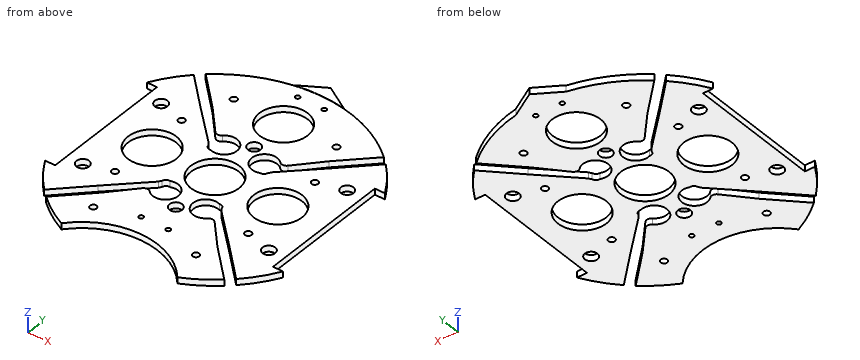
```python
from build123d import *

# Parameters (mm, degrees)
BOSS_EXTRUDE2_DEPTH      = 3.048
SKETCH4_R                = 38.1
CUT_EXTRUDE3_DEPTH       = 4.048
BOSS_EXTRUDE3_DEPTH      = 3.175
SKETCH12_R               = 1.143
CUT_EXTRUDE9_DEPTH       = 4.175
SKETCH15_R               = 1.651
CUT_EXTRUDE12_DEPTH      = 75.692
SKETCH17_R               = 1.651
CUT_EXTRUDE14_DEPTH      = 97.79
SKETCH18_R               = 12.192
CUT_EXTRUDE15_DEPTH      = 35.56
SKETCH19_R               = 3.175
CUT_EXTRUDE16_DEPTH      = 103.378
CUT_EXTRUDE16_DEPTH_BACK = 48.768
SKETCH5_R                = 12.192
CUT_EXTRUDE6_DEPTH       = 4.175
FILLET1_R                = 2.54
SKETCH20_R               = 1.143
CUT_EXTRUDE17_DEPTH      = 4.175


with BuildPart() as part:
    # Sketch1 → Boss-Extrude2 (new body)
    with BuildSketch(Plane.XY):
        with BuildLine():
            Line((-60.107370596, 33.02), (-55.027370596, 33.02))
            Line((-55.027370596, 33.02), (-55.027370596, -33.02))
            Line((-55.027370596, -33.02), (-60.107370596, -33.02))
            ThreePointArc((-60.107370596, -33.02), (0, -68.58), (60.107370596, -33.02))
            Line((60.107370596, -33.02), (55.027370596, -33.02))
            Line((55.027370596, -33.02), (55.027370596, 33.02))
            Line((55.027370596, 33.02), (60.107370596, 33.02))
            ThreePointArc((60.107370596, 33.02), (0, 68.58), (-60.107370596, 33.02))
        make_face()
    extrude(amount=BOSS_EXTRUDE2_DEPTH)

    # Sketch4 → Cut-Extrude3 (cut, through all)
    with BuildSketch(Plane(origin=(0, 0, 0), x_dir=(-1, 0, 0), z_dir=(0, 0, -1))):
        with Locations((0, -86.312058398)):
            Circle(SKETCH4_R)
    extrude(amount=-CUT_EXTRUDE3_DEPTH, mode=Mode.SUBTRACT)

    # Sketch9 → Boss-Extrude3 (add)
    with BuildSketch(Plane(origin=(0, 0, 0), x_dir=(-1, 0, 0), z_dir=(0, 0, -1))):
        with BuildLine():
            Line((12.7, 67.39381574), (0, 75))
            Line((0, 75), (-12.7, 67.39381574))
            ThreePointArc((-12.7, 67.39381574), (0, 68.58), (12.7, 67.39381574))
        make_face()
    extrude(amount=-BOSS_EXTRUDE3_DEPTH)

    # Sketch12 → Cut-Extrude9 (cut, through all)
    with BuildSketch(Plane(origin=(0, 0, 0), x_dir=(-1, 0, 0), z_dir=(0, 0, -1))):
        with Locations((6.731, 62.23)):
            Circle(SKETCH12_R)
        with Locations((-6.731, 62.23)):
            Circle(SKETCH12_R)
    extrude(amount=-CUT_EXTRUDE9_DEPTH, mode=Mode.SUBTRACT)

    # Sketch15 → Cut-Extrude12 (cut)
    with BuildSketch(Plane(origin=(30.092005081, 4.08352975, -3.048), x_dir=(-1, 0, 0), z_dir=(0, 0, -1))):
        with Locations((63.757223581, 17.50647025)):
            Circle(SKETCH15_R)
        with Locations((63.757223581, -25.67352975)):
            Circle(SKETCH15_R)
        with Locations((-3.552776419, -25.67352975)):
            Circle(SKETCH15_R)
        with Locations((-3.552776419, 17.50647025)):
            Circle(SKETCH15_R)
    extrude(amount=-CUT_EXTRUDE12_DEPTH, mode=Mode.SUBTRACT)

    # Sketch17 → Cut-Extrude14 (cut)
    with BuildSketch(Plane(origin=(30.092005081, 4.08352975, -33.0835), x_dir=(-1, 0, 0), z_dir=(0, 0, -1))):
        with Locations((4.154396091, -49.728759131)):
            Circle(SKETCH17_R)
        with Locations((56.02961407, -49.728759131)):
            Circle(SKETCH17_R)
        with Locations((4.154396091, 41.38247025)):
            Circle(SKETCH17_R)
        with Locations((56.02961407, 41.38247025)):
            Circle(SKETCH17_R)
    extrude(amount=-CUT_EXTRUDE14_DEPTH, mode=Mode.SUBTRACT)

    # Sketch18 → Cut-Extrude15 (cut)
    with BuildSketch(Plane(origin=(0, 0, 0), x_dir=(-1, 0, 0), z_dir=(0, 0, -1))):
        with Locations((31.75, 0)):
            Circle(SKETCH18_R)
        with Locations((-31.75, 0)):
            Circle(SKETCH18_R)
    extrude(amount=-CUT_EXTRUDE15_DEPTH, mode=Mode.SUBTRACT)

    # Sketch19 → Cut-Extrude16 (cut, two sides)
    with BuildSketch(Plane(origin=(30.092005081, 4.08352975, 3.048), x_dir=(-1, 0, 0), z_dir=(0, 0, -1))) as cut_extrude16_sk:
        with Locations((-16.897994919, 21.31647025)):
            Circle(SKETCH19_R)
        with Locations((77.082005081, 21.31647025)):
            Circle(SKETCH19_R)
        with Locations((30.092005081, 21.31647025)):
            Circle(SKETCH19_R)
        with Locations((77.082005081, -29.48352975)):
            Circle(SKETCH19_R)
        with Locations((30.092005081, -29.48352975)):
            Circle(SKETCH19_R)
        with Locations((-16.897994919, -29.48352975)):
            Circle(SKETCH19_R)
    extrude(amount=CUT_EXTRUDE16_DEPTH, mode=Mode.SUBTRACT)
    extrude(cut_extrude16_sk.sketch, amount=-CUT_EXTRUDE16_DEPTH_BACK, mode=Mode.SUBTRACT)

    # Sketch5 → Cut-Extrude6 (cut, through all)
    with BuildSketch(Plane(origin=(0, 0, 0), x_dir=(-1, 0, 0), z_dir=(0, 0, -1))):
        with BuildLine():
            Line((45.125787008, -51.860979099), (48.493383054, -48.493383054))
            Line((48.493383054, -48.493383054), (33.244765274, -33.244765274))
            Line((33.244765274, -33.244765274), (15.887580142, -16.296407899))
            ThreePointArc((15.887580142, -16.296407899), (15.502857332, -15.608744759), (15.036339126, -14.973722712))
            ThreePointArc((15.036339126, -14.973722712), (14.151046139, -13.510927072), (12.484618985, -13.128127778))
            ThreePointArc((12.484618985, -13.128127778), (4.300657145, -21.652046912), (16.112224352, -21.303752637))
            Line((16.112224352, -21.303752637), (29.410338797, -36.145530887))
            Line((29.410338797, -36.145530887), (45.125787008, -51.860979099))
        make_face()
        with BuildLine():
            ThreePointArc((15.036339126, 14.973722712), (15.502857332, 15.608744759), (15.887580142, 16.296407899))
            Line((15.887580142, 16.296407899), (33.244765274, 33.244765274))
            Line((33.244765274, 33.244765274), (48.493383054, 48.493383054))
            Line((48.493383054, 48.493383054), (45.125787008, 51.860979099))
            Line((45.125787008, 51.860979099), (29.410338797, 36.145530887))
            Line((29.410338797, 36.145530887), (16.112224352, 21.303752637))
            ThreePointArc((16.112224352, 21.303752637), (4.300657145, 21.652046912), (12.484618985, 13.128127778))
            ThreePointArc((12.484618985, 13.128127778), (14.151046139, 13.510927072), (15.036339126, 14.973722712))
        make_face()
        with BuildLine():
            ThreePointArc((-12.484618985, 13.128127778), (-4.300657145, 21.652046912), (-16.112224352, 21.303752637))
            Line((-16.112224352, 21.303752637), (-29.410338797, 36.145530887))
            Line((-29.410338797, 36.145530887), (-45.125787008, 51.860979099))
            Line((-45.125787008, 51.860979099), (-48.493383054, 48.493383054))
            Line((-48.493383054, 48.493383054), (-33.244765274, 33.244765274))
            Line((-33.244765274, 33.244765274), (-15.887580142, 16.296407899))
            ThreePointArc((-15.887580142, 16.296407899), (-15.502857332, 15.608744759), (-15.036339126, 14.973722712))
            ThreePointArc((-15.036339126, 14.973722712), (-14.151046139, 13.510927072), (-12.484618985, 13.128127778))
        make_face()
        with BuildLine():
            Line((-45.125787008, -51.860979099), (-29.410338797, -36.145530887))
            Line((-29.410338797, -36.145530887), (-16.112224352, -21.303752637))
            ThreePointArc((-16.112224352, -21.303752637), (-4.300657145, -21.652046912), (-12.484618985, -13.128127778))
            ThreePointArc((-12.484618985, -13.128127778), (-14.151046139, -13.510927072), (-15.036339126, -14.973722712))
            ThreePointArc((-15.036339126, -14.973722712), (-15.502857332, -15.608744759), (-15.887580142, -16.296407899))
            Line((-15.887580142, -16.296407899), (-33.244765274, -33.244765274))
            Line((-33.244765274, -33.244765274), (-48.493383054, -48.493383054))
            Line((-48.493383054, -48.493383054), (-45.125787008, -51.860979099))
        make_face()
        Circle(SKETCH5_R)
        with Locations((0, 44.45)):
            Circle(SKETCH5_R)
    extrude(amount=-CUT_EXTRUDE6_DEPTH, mode=Mode.SUBTRACT)

    # Fillet1
    fillet1_edges = [part.edges().sort_by_distance(p)[0] for p in [
        (-16.112224352, -21.303752637, 1.524),
        (-16.112224352, 21.303752637, 1.524),
        (16.112224352, 21.303752637, 1.524),
        (16.112224352, -21.303752637, 1.524),
    ]]
    fillet(fillet1_edges, radius=FILLET1_R)

    # Sketch20 → Cut-Extrude17 (cut, through all)
    with BuildSketch(Plane(origin=(0, 0, 0), x_dir=(-1, 0, 0), z_dir=(0, 0, -1))):
        with Locations((-6.858, -39.116)):
            Circle(SKETCH20_R)
        with Locations((6.858, -39.116)):
            Circle(SKETCH20_R)
    extrude(amount=-CUT_EXTRUDE17_DEPTH, mode=Mode.SUBTRACT)


solid = part.part
```
For this review, take the finished solid that the model builds, in its own axes (mm). Round coordinates to 2 decimals unless told otherwise and drop trailing zeros. Write each loop counter-clockwise with the first axis right and the second up, starting at its lowest first coordinate (ties: lowest second). Pieces come first, ordered by that corner, then holes. Notation, with made-up numbers: (-10.5, 35.5) -> (14.5, 35.5) arc R19 ccw to (14.5, 49.5) -> close; hole circle Ø8 at (10.5, -23.5). An arc over 180 degrees is marked (long way). Use one line per item in the form item = value.
Q1. Consider section B-B (x = -46.99). State the section outline as (y, z) points (3 decimals).
Resolved:
outline = (-46.99, 0) -> (-28.575, 0) -> (-28.575, 3.048) -> (-46.99, 3.048) -> close; (-22.225, 0) -> (22.225, 0) -> (22.225, 3.048) -> (-22.225, 3.048) -> close; (28.575, 0) -> (46.99, 0) -> (46.99, 3.048) -> (28.575, 3.048) -> close
Q2. Clearance check with flat-ended pins moving along their axes: pin 1 Ø4 at (x, y) = (-25.94, 45.47) entering from +Z; pin 2 Ø14.5 at (x, y) = (0, 44.45) entering from -Z. State where each tip first meets the part, or that it passes through.
Resolved:
pin_1 = 3.05
pin_2 = through
Q3. Consider section C-C (y = -42). State the section outline as (x, z) points, then the cut area to 3 significant figures.
Resolved:
outline = (-54.21, 0) -> (-42, 0) -> (-42, 3.05) -> (-54.21, 3.05) -> close; (-35.26, 0) -> (35.26, 0) -> (35.26, 3.05) -> (-35.26, 3.05) -> close; (42, 0) -> (54.21, 0) -> (54.21, 3.05) -> (42, 3.05) -> close
area = 289 mm²
Q4. Consider section D-D (x = 40.5). State the section outline as (y, z) points.
Resolved:
outline = (-55.34, 0) -> (-47.24, 0) -> (-47.24, 3.05) -> (-55.34, 3.05) -> close; (-40.5, 0) -> (-8.49, 0) -> (-8.49, 3.05) -> (-40.5, 3.05) -> close; (8.49, 0) -> (40.5, 0) -> (40.5, 3.05) -> (8.49, 3.05) -> close; (47.24, 0) -> (55.34, 0) -> (55.34, 3.05) -> (47.24, 3.05) -> close
Q5. To check wall thickness, follow probe 1 along X at (y, z) = (29, 2.65); probe 2 along X at (y, z) = (8, 2.9); probe 3 along X at (y, z) = (31.5, 1.4). State the ranges of each line that lie inside material, in increasing order. Write a range as from..to.
Resolved:
probe_1 = -55.03..-28.9, -23.01..23.01, 28.9..55.03
probe_2 = -55.03..-40.95, -22.55..-9.2, 9.2..22.55, 40.95..55.03
probe_3 = -55.03..-31.46, -25.25..25.25, 31.46..55.03
Q6. Consider section A-A (y = 0). State the section outline as (x, z) points.
Resolved:
outline = (-55.03, 0) -> (-43.94, 0) -> (-43.94, 3.05) -> (-55.03, 3.05) -> close; (-19.56, 0) -> (-12.19, 0) -> (-12.19, 3.05) -> (-19.56, 3.05) -> close; (12.19, 0) -> (19.56, 0) -> (19.56, 3.05) -> (12.19, 3.05) -> close; (43.94, 0) -> (55.03, 0) -> (55.03, 3.05) -> (43.94, 3.05) -> close
